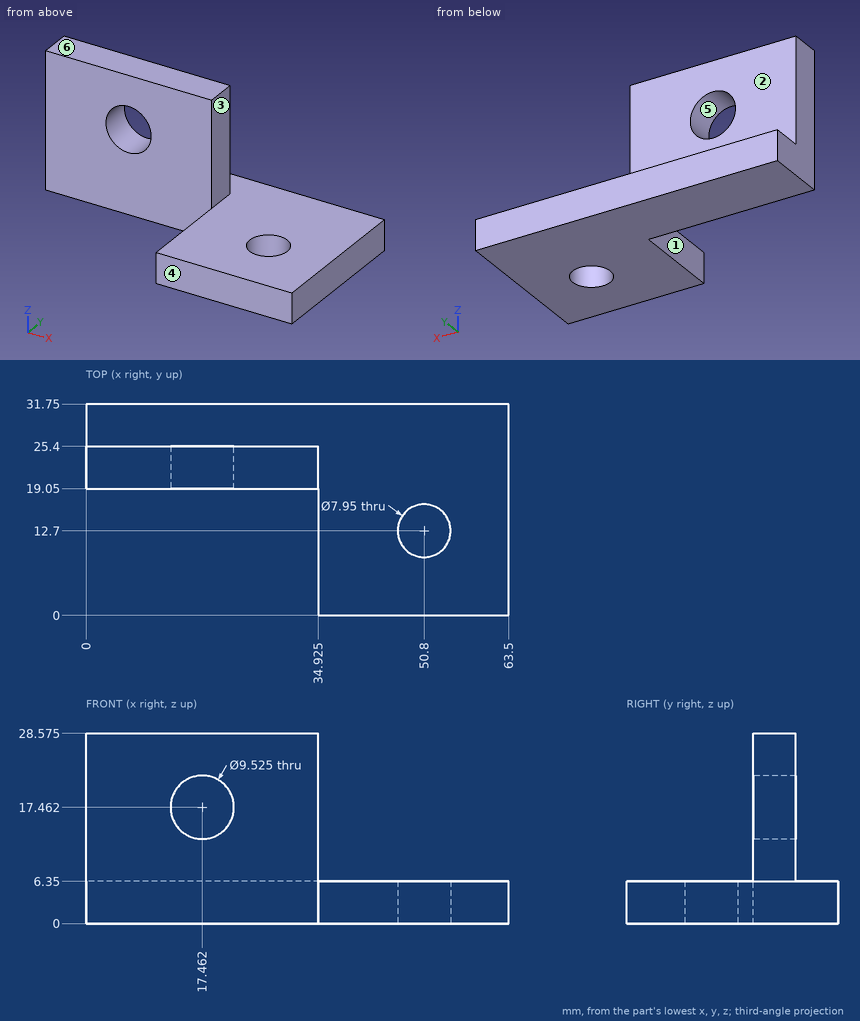
Study the drawing (mm; zero at the part's minimum x, y, z) and answer. A direction names the side the tool comes from. Give positions to 0.01 mm unless a question says otherwise; leave off trailing zeros. Use one line per item in the form item = value. Start each with the question number.
(1) For the marked faces 1, 2 and 3, determine the directions among +Z, -Z, +X, -X, +Y, -Y from which every point of the face is accessible in a straight line to the end or side of a thin tool.
(2) The mould has two halves that part along Z. Classify the marked faces 4, 5 and 6: released by +Z, released by -Z, zero draft, split by the parting line, or undercut.
(3) Flat-ended cylindrical pins translate along their axes: pin 1 Ø5 at (y, z) = (14, 1.5) entering from -X (1 decimal); pin 2 Ø3 at (y, z) = (23.5, 18.5) entering from +X (1 decimal); pin 3 Ø3 at (x, y) = (49.5, 23) entering from +Z. Find the tip coordinate at first contact, or state that the pin passes through.
(4) Consider line 1 (X direction, y = 13, z = 1.5) (1 decimal); line 2 (Y direction, x = 14.5, z = 3.25); line 3 (Z direction, x = 37.5, y = 22). Determine where each line is inside the solid, lowest interval first. Write a range as from..to.
Ans:
q1.face_1 = +Z, -Z, -X, -Y
q1.face_2 = +Z, +X, -X, +Y
q1.face_3 = +Z, +X, +Y, -Y
q2.face_4 = zero draft
q2.face_5 = undercut
q2.face_6 = released by +Z
q3.pin_1 = 34.9
q3.pin_2 = 34.9
q3.pin_3 = 6.35
q4.line_1 = 34.9..46.8, 54.8..63.5
q4.line_2 = 19.05..31.75
q4.line_3 = 0..6.35
